Read the model definition and answer for the solid it produces. Units are mm, in the model's axes. Face numbers are marked on the shaded views. A direction names the side the tool comes from. Coordinates: 2 decimals unless noted, no trailing zeros. Loops run counter-clockwise (first coordinate to the right, second up) from the corner with the lowest first, then second, coordinate; pieces in that order, holes last. Notation, with made-up numbers: (76.25, 56.5) -> (81.25, 56.5) arc R13 cw to (81.25, 61.5) -> close; hole circle Ø6 at (24.25, 60). An arc over 180 degrees is marked (long way). Answer as a JSON object with one key per item and string values. Group by question number.
1) Determine the mould class of the marked faces 5, 6 and 7 for opening direction Y: released by +Y, released by -Y, zero draft, split by the parting line, or undercut.
2) Flat-ended cylindrical pins translate along their axes: P1, Ø9, axis at y = 21, z = 13, coming from the -X side; P2, Ø6, axis at x = -22, y = -20.5, coming from the +Z side; P3, Ø5, axis at x = 19.5, z = -14.5, coming from the -Y side. Find the tip coordinate at first contact, or state that the pin passes through.
3) Which of the six approach directions +Z, -Z, +X, -X, +Y, -Y give full straight-line access (tool end or side, diameter ignored) to the marked faces 1, 2, 3 and 4?
4) Section C-C, the plane y = 60 is taken. Give the vertices of the cut face in (x, z), plus the area to 3 significant figures.
5) Section A-A, the plane x = 0 is taken. Give the vertices of the cut face in (y, z), plus the area to 3 significant figures.
6) Section B-B, the plane y = 24 is taken. Give the vertices of the cut face in (x, z), plus the area to 3 significant figures.
7) Consider probe 1 along Y at (x, z) = (-15, 29); probe 2 along Y at (x, z) = (24.5, -19); probe 3 along Z at (x, y) = (25, 59.5). Determine where each line is inside the solid, lowest interval first. Write a range as [from, to].
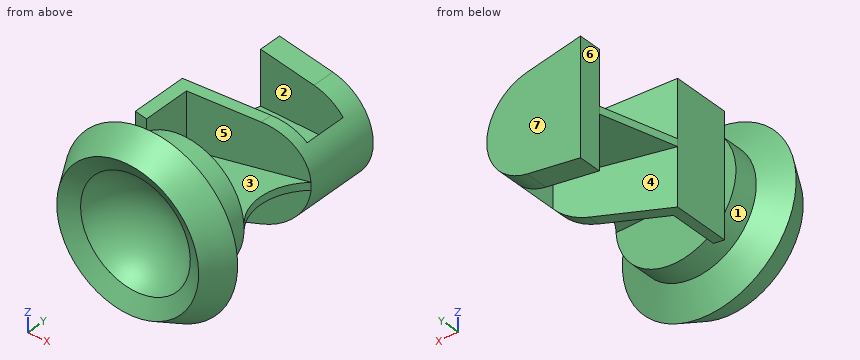
from build123d import *

# Parameters (mm, degrees)
BOSS_EXTRUDE1_DEPTH = 40
RIB7_START          = -2
RIB7_DEPTH          = 4
SKETCH2_OUTSIDE_W   = 129.678
SKETCH2_OUTSIDE_H   = 129.678
CUT_EXTRUDE1_DEPTH  = 80
RIB1_REACH          = 105.413
SKETCH3_WALL_W      = 248.119937824
SKETCH3_WALL_H      = 4


# Read off the part's stored shape, not the designer's step: Rib7
with BuildPart() as part:
    # Sketch1 → Revolve1 (revolve)
    with BuildSketch(Plane.XY, mode=Mode.PRIVATE) as revolve1_sk:
        with BuildLine():
            Line((-37.837168574, -36), (-29.262233414, -31.049258877))
            ThreePointArc((-29.262233414, -31.049258877), (-17.458182667, -17.181874451), (0, -12))
            Line((0, -12), (0, 0))
            Line((0, 0), (-32, 0))
            Line((-32, 0), (-32, -13))
            Line((-32, -13), (-46.337168574, -21.277568136))
            Line((-46.337168574, -21.277568136), (-37.837168574, -36))
        make_face()
    revolve(revolve1_sk.sketch.rotate(Axis((0, 0, 0), (0, -1, 0)), 270), axis=Axis((0, 0, 0), (0, -1, 0)))

    # Sketch1<3> → Boss-Extrude1 (add, symmetric)
    with BuildSketch(Plane.XY):
        Polygon((-26, 0), (-20, 0), (-20, 25.439486103), (34, 40.439486103), (34, 80), (-16, 80), (-16, 68), (28, 68), (28, 45), (-26, 30), align=None)
    extrude(amount=BOSS_EXTRUDE1_DEPTH, both=True)

    # Rib7 outline → Rib7 (add)
    with BuildSketch(Plane.XY.offset(RIB7_START)):
        with BuildLine():
            Line((-20, 0), (32, 0))
            ThreePointArc((32, 0), (24.570511929, 20.636636978), (34, 40.439486103))
            Line((34, 40.439486103), (-20, 25.439486103))
            Line((-20, 25.439486103), (-20, 0))
        make_face()
    extrude(amount=RIB7_DEPTH)

    # Sketch2 outside → Cut-Extrude1 (cut)
    with BuildSketch(Plane(origin=(0, 80, 0), x_dir=(1, 0, 0), z_dir=(0, 1, 0))):
        Rectangle(SKETCH2_OUTSIDE_W, SKETCH2_OUTSIDE_H)
        with BuildLine():
            Line((12.412638687, 25.726815399), (-26, 32.5))
            Line((-26, 32.5), (-26, -32.5))
            Line((-26, -32.5), (12.412638687, -25.726815399))
            ThreePointArc((12.412638687, -25.726815399), (34, 0), (12.412638687, 25.726815399))
        make_face(mode=Mode.SUBTRACT)
    extrude(amount=-CUT_EXTRUDE1_DEPTH, mode=Mode.SUBTRACT)

    # Sketch3 wall → Rib1 (add, up to next)
    with BuildSketch(Plane(origin=(-21, 49, 0), x_dir=(-0.25449329928, -0.967074537263, 0), z_dir=(0.967074537263, -0.25449329928, 0)), mode=Mode.PRIVATE) as rib1_sk1:
        Rectangle(SKETCH3_WALL_W, SKETCH3_WALL_H)
    rib1_tool1 = extrude(rib1_sk1.sketch, amount=RIB1_REACH, mode=Mode.PRIVATE) - part.part
    add(rib1_tool1.solids().sort_by_distance((-21, 49, 0))[0])


solid = part.part
Determined:
{
 "1": {"face 5": "undercut", "face 6": "zero draft", "face 7": "released by +Y"},
 "2": {"P1": "x = -26", "P2": "z = 42.22", "P3": "y = -26.51"},
 "3": {"face 1": "none", "face 2": "+Z, -X", "face 3": "+Z, +X", "face 4": "-Z, -X"},
 "4": {"outline": "(-18.11, -2) -> (28, -2) -> (28, -16.66) arc R26.12 ccw to (28, 16.66) -> (28, 2) -> (-18.11, 2) -> close", "area": "321 mm²"},
 "5": {"outline": "(-36, -37.84) -> (-21.28, -46.34) -> (-13, -32) -> (0, -32) -> (0, -2) -> (31, -2) -> (31, -27.92) -> (37.22, -27.92) -> (37.22, -2) -> (68, -2) -> (68, -27.92) -> (80, -27.92) -> (80, 27.92) -> (68, 27.92) -> (68, 2) -> (37.22, 2) -> (37.22, 27.92) -> (31, 27.92) -> (31, 2) -> (0, 2) -> (0, 32) -> (-13, 32) -> (-21.28, 46.34) -> (-36, 37.84) -> (-31.05, 29.26) arc R32 cw to (-31.05, -29.26) -> close", "area": "2,850 mm²"},
 "6": {"outline": "(-26, -32.5) -> (-20, -31.44) -> (-20, -2) -> (24.94, -2) -> (24.94, 2) -> (-20, 2) -> (-20, 31.44) -> (-26, 32.5) -> close", "area": "563 mm²"},
 "7": {"probe 1": "[-33, -13.38], [26.83, 33.06], [68, 80]", "probe 2": "[-32.05, 0], [37.8, 44.03], [68, 80]", "probe 3": "[-2, 2]"}
}
